from build123d import *

# Parameters (mm, degrees)
SKETCH1_W             = 30
SKETCH1_H             = 35
BOSS_EXTRUDE1_DEPTH   = 5
SKETCH1_3_W           = 5
SKETCH1_3_H           = 35
BOSS_EXTRUDE2_DEPTH   = 20
CUT_EXTRUDE1_DEPTH    = 5
CUT_EXTRUDE2_DEPTH    = 3.8
SKETCH3_R             = 2.151
BOSS_EXTRUDE3_DEPTH   = 5.4
RIB1_START            = -1
RIB1_DEPTH            = 2
CIRPATTERN6_COUNT     = 4
SKETCH6_W             = 5.4
SKETCH6_H             = 0.862
BOSS_EXTRUDE4_DEPTH   = 1
MIRROR1_START         = -1
MIRROR1_COPY_1_DEPTH  = 2
MIRROR1_COPY_2_DEPTH  = 2
M2_TAPPED_HOLE1_D     = 1.6
M2_TAPPED_HOLE1_DEPTH = 5.4
M2_TAPPED_HOLE1_TIP   = 0.480688495


with BuildPart() as part:
    # Sketch1 → Boss-Extrude1 (new body)
    with BuildSketch(Plane(origin=(0, 0, 0), x_dir=(1, 0, 0), z_dir=(0, 1, 0))):
        with Locations((20, 17.5)):
            Rectangle(SKETCH1_W, SKETCH1_H)
    extrude(amount=BOSS_EXTRUDE1_DEPTH)

    # Sketch1<3> → Boss-Extrude2 (add)
    with BuildSketch(Plane(origin=(0, 0, 0), x_dir=(1, 0, 0), z_dir=(0, 1, 0))):
        with Locations((2.5, 17.5)):
            Rectangle(SKETCH1_3_W, SKETCH1_3_H)
    extrude(amount=BOSS_EXTRUDE2_DEPTH)

    # Sketch2 → Cut-Extrude1 (cut)
    with BuildSketch(Plane.ZY):
        with BuildLine():
            Line((-20.3, 12), (-14.7, 12))
            ThreePointArc((-14.7, 12), (-12.95, 13.75), (-14.7, 15.5))
            Line((-14.7, 15.5), (-20.3, 15.5))
            ThreePointArc((-20.3, 15.5), (-22.05, 13.75), (-20.3, 12))
        make_face()
    extrude(amount=-CUT_EXTRUDE1_DEPTH, mode=Mode.SUBTRACT)

    # Sketch2<4> → Cut-Extrude2 (cut)
    with BuildSketch(Plane.ZY):
        with BuildLine():
            Line((-20.3, 18.5), (-14.7, 18.5))
            ThreePointArc((-14.7, 18.5), (-9.95, 13.75), (-14.7, 9))
            Line((-14.7, 9), (-20.3, 9))
            ThreePointArc((-20.3, 9), (-25.05, 13.75), (-20.3, 18.5))
        make_face()
        with BuildLine():
            ThreePointArc((-14.7, 12), (-12.95, 13.75), (-14.7, 15.5))
            Line((-14.7, 15.5), (-20.3, 15.5))
            ThreePointArc((-20.3, 15.5), (-22.05, 13.75), (-20.3, 12))
            Line((-20.3, 12), (-14.7, 12))
        make_face(mode=Mode.SUBTRACT)
    extrude(amount=-CUT_EXTRUDE2_DEPTH, mode=Mode.SUBTRACT)

    # Sketch3 → Boss-Extrude3 (add)
    with BuildSketch(Plane(origin=(0, 5, 0), x_dir=(1, 0, 0), z_dir=(0, 1, 0))):
        with Locations(Location((7.513, 25.755, 0), (0, 0, 90))):
            Circle(SKETCH3_R)
        with Locations(Location((7.513, 9.245, 0), (0, 0, 90))):
            Circle(SKETCH3_R)
    extrude(amount=BOSS_EXTRUDE3_DEPTH)

    # Rib1: read off the stored shape, not the designer's step
    # Rib1 outline → Rib1 (add)
    with BuildSketch(Plane(origin=(7.513, 0, 0), x_dir=(0, 0, -1), z_dir=(1, 0, 0)).offset(RIB1_START)):
        Polygon((7.094, 10.4), (4.094, 5), (7.340583816, 5), (7.340583816, 10.4), align=None)
    rib1 = extrude(amount=RIB1_DEPTH)

    # CirPattern6: Rib1 ×4 about axis, 1 skipped
    cirpattern6_axis = Axis((7.513, 0, -9.245), (0, 1, 0))
    add([rib1.rotate(cirpattern6_axis, i * 360 / CIRPATTERN6_COUNT) for i in range(1, CIRPATTERN6_COUNT) if i not in (3,)])

    # Sketch6 → Boss-Extrude4 (add, symmetric)
    with BuildSketch(Plane(origin=(0, 0, -9.245), x_dir=(0, -1, 0), z_dir=(0, 0, 1))):
        with Locations((-7.7, 5.431)):
            Rectangle(SKETCH6_W, SKETCH6_H)
    boss_extrude4 = extrude(amount=BOSS_EXTRUDE4_DEPTH, both=True)

    # Mirror1: Rib1, Boss-Extrude4 across plane
    add(rib1.mirror(Plane.XY.offset(-17.5)))
    add(boss_extrude4.mirror(Plane.XY.offset(-17.5)))

    # Mirror1 copy 1 sketch → Mirror1 copy 1 (add)
    with BuildSketch(Plane(origin=(16.758, 0, -25.755), x_dir=(-1, 0, 0), z_dir=(0, 0, 1)).offset(MIRROR1_START)):
        Polygon((7.094, -10.4), (4.094, -5), (7.340583816, -5), (7.340583816, -10.4), align=None)
    extrude(amount=MIRROR1_COPY_1_DEPTH)

    # Mirror1 copy 2 sketch → Mirror1 copy 2 (add)
    with BuildSketch(Plane(origin=(7.513, 0, -16.51), x_dir=(0, 0, -1), z_dir=(-1, 0, 0)).offset(MIRROR1_START)):
        Polygon((7.094, -10.4), (4.094, -5), (7.340583816, -5), (7.340583816, -10.4), align=None)
    extrude(amount=MIRROR1_COPY_2_DEPTH)

    # M2 Tapped Hole1
    with Locations(Plane(origin=(0, 10.4, 0), x_dir=(1, 0, 0), z_dir=(0, 1, 0))):
        with Locations((7.513, 9.245), (7.513, 25.755)):
            Hole(M2_TAPPED_HOLE1_D / 2, depth=M2_TAPPED_HOLE1_DEPTH)
            with Locations((0, 0, -(M2_TAPPED_HOLE1_DEPTH + M2_TAPPED_HOLE1_TIP / 2))):  # 118° drill point
                Cone(0, M2_TAPPED_HOLE1_D / 2, M2_TAPPED_HOLE1_TIP, mode=Mode.SUBTRACT)


solid = part.part
Check sheet for the modelled part. Datum: model origin and axes. Units: mm. A direction names the side the tool comes from. Round coordinates to 2 decimals unless told otherwise and drop trailing zeros. Order: outer loops, then holes, each group sorted by start corner. A loop starts at its lowest first (then second) coordinate and runs counter-clockwise, first axis right, second up.
Q1. Depth check by flat-ended pin: P1, Ø1.3, axis at x = 7, z = -10, coming from the +Y side; P2, Ø0.5, axis at x = 5.5, y = 7, coming from the -Z side; P3, Ø1.6, axis at x = 11.5, y = 7.5, coming from the -Z side (3 decimals). Enter the tip coordinate at first touch or a pass-through.
Filled sheet:
P1: stops at y = 10.4
P2: stops at z = -26.99
P3: stops at z = -26.755
Q2. Cross-section at B-B, the plane z = -18.5. Enter the section's corners in (x, y), plus the area to 3 significant figures.
Filled sheet:
outline: (0, 0) - (35, 0) - (35, 5) - (5, 5) - (5, 12) - (3.8, 12) - (3.8, 9) - (0, 9) - close; (0, 18.5) - (3.8, 18.5) - (3.8, 15.5) - (5, 15.5) - (5, 20) - (0, 20) - close
area: 210 mm2
Q3. Scan lines: L1, parallel to X at y = 7.25, z = -12; L2, parallel to X at y = 16.5, z = -23; L3, parallel to X at y = 17, z = -26. Record each from-to range of solid material in increasing order.
Filled sheet:
L1: x = 0 to 5, 6.51 to 8.51
L2: x = 3.8 to 5
L3: x = 0 to 5
Q4. Cross-section at A-A, the plane y = 13.75. Enter the section's corners in (x, z), plus the area to 3 significant figures.
Filled sheet:
outline: (0, -35) - (5, -35) - (5, -22.05) - (3.8, -22.05) - (3.8, -25.05) - (0, -25.05) - close; (0, -9.95) - (3.8, -9.95) - (3.8, -12.95) - (5, -12.95) - (5, 0) - (0, 0) - close
area: 107 mm2
Q5. Draft check along X on faces 1 (the face through (7.641, 4.603, -9.192)), 2 (the face through (3.8, 11.7, -17.4)), 3 (the face through (11.14, 7.74, -9.23)). Enter one of: pulls with the +X half, pulls with the -X half, needs draft (parallel to the pull), parting line crosses it, or undercut.
Filled sheet:
face 1: undercut
face 2: pulls with the -X half
face 3: pulls with the +X half
Q6. Cross-section at D-D, the plane y = 17.5. Enter the section's corners in (x, z), plus the area to 3 significant figures.
Filled sheet:
outline: (0, -35) - (5, -35) - (5, 0) - (0, 0) - (0, -11.78) - (3.8, -11.78) - (3.8, -23.22) - (0, -23.22) - close
area: 132 mm2
Q7. Set-up check for faces 4 (the face through (10, 7, -10.245)), 5 (the face through (2, 18.5, -18)), 6 (the face through (6.513, 7, -23)): record each of +Z, -Z, +X, -X, +Y, -Y from which the full face is reachable in a straight line by a thin tool's end or side.
Filled sheet:
face 4: +X, +Y
face 5: -X
face 6: +Y
Q8. Cross-section at C-C, the plane x = 3. Enter the section's corners in (y, z).
Filled sheet:
outline: (0, -35) - (20, -35) - (20, 0) - (0, 0) - close; hole (9, -20.3) arc R4.75 ccw to (18.5, -20.3) - (18.5, -14.7) arc R4.75 ccw to (9, -14.7) - close
